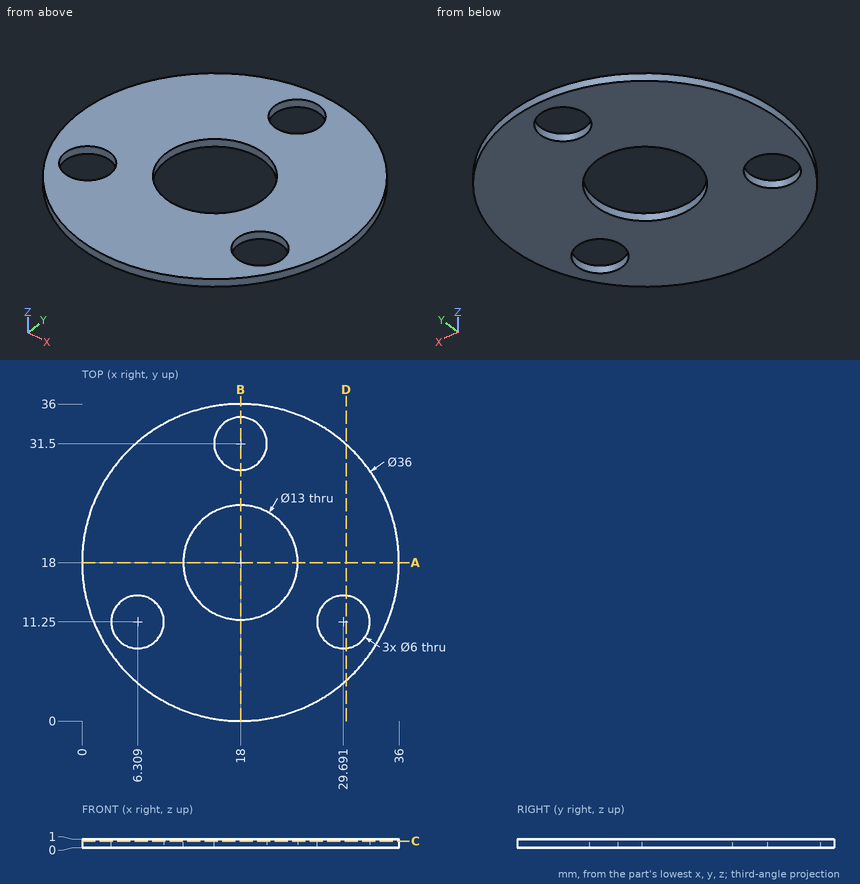
Geometry check sheet. Reference: drawing and pictorial views, mm from the part's lowest x, y, z. Give positions to 0.01 mm unless a question says otherwise; leave off trailing zeros. Order: outer loops, then holes, each group sorted by start corner. A loop starts at its lowest first (then second) coordinate and runs counter-clockwise, first axis right, second up. Notation, with made-up numbers: M -2,48.5 L 15,48.5 A20 cw 15,63.5 Z; hole C -1,54.5 d9. An arc over 180 degrees is marked long. Return JSON: item names as keys, results as strings. Group by question number.
1) Section check A-A on y = 18. Record the cut outline in (x, z).
2) Section check B-B on x = 18. Record the cut outline in (y, z).
3) Section check D-D on x = 30. Record the cut outline in (y, z).
4) Section check C-C on z = 0.75. Record the cut outline in (x, y).
5) Scan lines: line 1 (Y direction, x = 18, z = 0.75); line 2 (X direction, y = 9.5, z = 0.9) (1 decimal); line 3 (Y direction, x = 17, z = 0.8). Record each from-to range of solid material in increasing order.
Answer block:
{
 "1": {"outline": "M 0,0 L 11.5,0 L 11.5,1 L 0,1 Z; M 24.5,0 L 36,0 L 36,1 L 24.5,1 Z"},
 "2": {"outline": "M 0,0 L 11.5,0 L 11.5,1 L 0,1 Z; M 24.5,0 L 28.5,0 L 28.5,1 L 24.5,1 Z; M 34.5,0 L 36,0 L 36,1 L 34.5,1 Z"},
 "3": {"outline": "M 4.58,0 L 8.27,0 L 8.27,1 L 4.58,1 Z; M 14.23,0 L 31.42,0 L 31.42,1 L 14.23,1 Z"},
 "4": {"outline": "C 18,18 d36; hole C 6.31,11.25 d6; hole C 18,18 d13; hole C 18,31.5 d6; hole C 29.69,11.25 d6"},
 "5": {"line 1": "y = 0 to 11.5, 24.5 to 28.5, 34.5 to 36", "line 2": "x = 2.1 to 3.9, 8.7 to 27.3, 32.1 to 33.9", "line 3": "y = 0.03 to 11.58, 24.42 to 28.67, 34.33 to 35.97"}
}
